Input: part model. Units: mm. Frame: model coordinates. A direction names the side the tool comes from. Coordinates: 2 decimals unless noted, no trailing zeros. Loops run counter-clockwise (first coordinate to the right, second up) from the corner with the lowest first, then second, coordinate; pieces in that order, holes last. Notation, with made-up numbers: (-22, 1.5) -> (-9, 1.5) arc R11 ccw to (-9, 6.5) -> close; hole circle Ø9 at (23, -5.75). An arc over 180 degrees is marked (long way). Put each result on its own line as item: value. Start each with the question number.
1) Cut plane A-A (y = 0). Return the cut outline in (x, z), plus the area to 3 significant figures.
2) Set-up query: faces 1 (the cylindrical face through (55.431, -42.503, 15.742)), 2 (the flat face through (-1, 1, 0)). Return all of +Z, -Z, +X, -X, +Y, -Y with unobstructed straight access to the full face (end or side cutting, diameter ignored); none if empty.
3) Contact query for flat-ended pins moving along their axis: P1, Ø3, axis at y = -9.5, z = 19, coming from the -X side; P2, Ø1, axis at x = 38.5, z = 10.5, coming from the +Y side; P3, Ø10, axis at x = -4.5, y = 24, coming from the +Z side. Output: stop coordinate, or through.
4) Material intervals for L1, parallel to Y at x = 0, z = 10.5; L2, parallel to Z at x = -34, y = -13.5; L3, parallel to X at y = 22.5, z = 24, sorted ascending.
5) Cut plane C-C (z = 20.5). Return the cut outline in (x, y).
from build123d import *

# Parameters (mm, degrees)
F0_R     = 76.2
F1_DEPTH = 25.4
F2_SIZE  = 5.08
F4_D     = 139.7
F5_R     = 69.85
F6_DEPTH = 6.35


with BuildPart() as f1:
    # F0 (on Top) → F1 (new body)
    with BuildSketch(Plane.XY):
        Circle(F0_R)
    extrude(amount=F1_DEPTH)

    # F2
    f2_edges = [f1.edges().sort_by_distance(p)[0] for p in [
        (-76.2, 0, 0),
    ]]
    chamfer(f2_edges, length=F2_SIZE)

    # F4 (through all)
    with Locations(Plane.XY.offset(25.4)):
        with Locations((0, 0)):
            Hole(F4_D / 2)

    # F5 (on Top) → F6 (join)
    with BuildSketch(Plane.XY):
        Circle(F5_R)
    extrude(amount=F6_DEPTH)


solid = f1.part
Results found:
1. outline: (-76.2, 5.08) -> (-71.12, 0) -> (71.12, 0) -> (76.2, 5.08) -> (76.2, 25.4) -> (69.85, 25.4) -> (69.85, 6.35) -> (-69.85, 6.35) -> (-69.85, 25.4) -> (-76.2, 25.4) -> close
1. area: 1,180 mm2
2. face 1: +Z
2. face 2: -Z, +X, -X, +Y, -Y
3. P1: stops at x = -75.78
3. P2: stops at y = 66.05
3. P3: stops at z = 6.35
4. L1: y = -76.2 to -69.85, 69.85 to 76.2
4. L2: z = 0 to 6.35
4. L3: x = -72.8 to -66.13, 66.13 to 72.8
5. outline: circle Ø152.4 at (0, 0); hole circle Ø139.7 at (0, 0)
